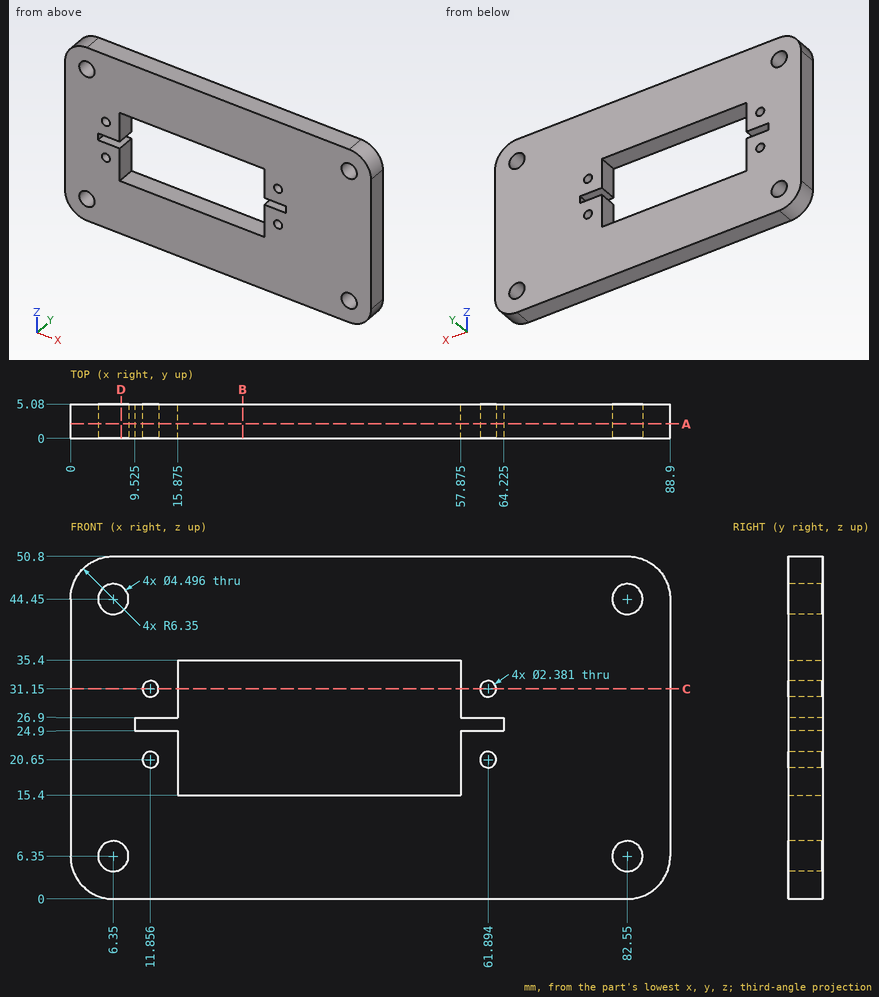
Verification items for this drawing (mm, ordinates from the low corner). Give positions to 0.01 mm unless a question says otherwise; leave off trailing zeros. Write each loop counter-clockwise with the first axis right and the second up, starting at its lowest first coordinate (ties: lowest second). Pieces come first, ordered by that corner, then holes.
1) Section check C-C, the plane z = 31.15. Record the boundary of the cut face in (x, y) (1 decimal), and give its area (3 significant figures).
2) Section check A-A, the plane y = 2.15. State how many separate pieces and enclosed holes the cut face has, and give its area (4 significant figures).
3) Material ranges on L1, parallel to Z at x = 6.35, y = 2.4; L2, parallel to X at y = 1.15, z = 44.45; L3, parallel to X at y = 1.7, z = 20.65 (1 decimal), recorded low to high.
4) Section check D-D, the plane x = 7.5. Record the boundary of the cut face in (y, z), and give its area (3 significant figures).
5) Section check B-B, the plane x = 25.5. Record the boundary of the cut face in (y, z).
6) Gauge pin test, flat end, axial feed: pin 1 (12 mm diameter, centred on x = 38, z = 35.5, fed in from -Y). Record the tip position at first contact, or that the pin passes through.
Computed:
1. outline: (0, 0) - (10.7, 0) - (10.7, 5.1) - (0, 5.1) - close; (13, 0) - (15.9, 0) - (15.9, 5.1) - (13, 5.1) - close; (57.9, 0) - (60.7, 0) - (60.7, 5.1) - (57.9, 5.1) - close; (63.1, 0) - (88.9, 0) - (88.9, 5.1) - (63.1, 5.1) - close
1. area: 214 mm2
2. separate pieces: 1
2. enclosed holes: 9
2. area: 3,535 mm2
3. L1: z = 0 to 4.1, 8.6 to 42.2, 46.7 to 50.8
3. L2: x = 0 to 4.1, 8.6 to 80.3, 84.8 to 88.9
3. L3: x = 0 to 10.7, 13 to 15.9, 57.9 to 60.7, 63.1 to 88.9
4. outline: (0, 0) - (5.08, 0) - (5.08, 4.42) - (0, 4.42) - close; (0, 8.28) - (5.08, 8.28) - (5.08, 42.52) - (0, 42.52) - close; (0, 46.38) - (5.08, 46.38) - (5.08, 50.8) - (0, 50.8) - close
4. area: 219 mm2
5. outline: (0, 0) - (5.08, 0) - (5.08, 15.4) - (0, 15.4) - close; (0, 35.4) - (5.08, 35.4) - (5.08, 50.8) - (0, 50.8) - close
6. pin 1: stops at y = 0
